Here's how the part is built. I have some questions about the finished solid (model axes, mm). A direction names the side the tool comes from. Give positions to 0.01 mm unless a question says otherwise; leave off trailing zeros. Loops run counter-clockwise (first coordinate to the right, second up) from the corner with the lowest first, then second, coordinate; pieces in that order, holes last. Notation, with made-up numbers: (36, 12) - (87, 12) arc R28 ccw to (87, 34) - close; hole circle Ø5 at (73.25, 73). An arc over 180 degrees is marked (long way). Use a Markdown table: item, result.
from build123d import *

# Parameters (mm, degrees)
F1_DEPTH = 5


with BuildPart() as f1:
    # F0 (on Front) → F1 (new body)
    with BuildSketch(Plane.XZ):
        with BuildLine():
            ThreePointArc((40, 105), (37.071068, 112.071068), (30, 115))
            Line((30, 115), (-30, 115))
            ThreePointArc((-30, 115), (-37.071068, 112.071068), (-40, 105))
            Line((-40, 105), (-40, 97.5))
            Line((-40, 97.5), (-33, 97.5))
            ThreePointArc((-33, 97.5), (-27.87868, 99.62132), (-30, 94.5))
            Line((-30, 94.5), (-30, -94.5))
            ThreePointArc((-30, -94.5), (-27.87868, -99.62132), (-33, -97.5))
            Line((-33, -97.5), (-40, -97.5))
            Line((-40, -97.5), (-40, -105))
            ThreePointArc((-40, -105), (-37.071068, -112.071068), (-30, -115))
            Line((-30, -115), (30, -115))
            ThreePointArc((30, -115), (37.071068, -112.071068), (40, -105))
            Line((40, -105), (40, -97.5))
            Line((40, -97.5), (33, -97.5))
            ThreePointArc((33, -97.5), (27.87868, -99.62132), (30, -94.5))
            Line((30, -94.5), (30, 94.5))
            ThreePointArc((30, 94.5), (27.87868, 99.62132), (33, 97.5))
            Line((33, 97.5), (40, 97.5))
            Line((40, 97.5), (40, 105))
        make_face()
    extrude(amount=F1_DEPTH)


solid = f1.part
(1) We'd pull the mould along X, two halves only. Please class faces 1 (the face through (27.95, -2.46, -99.69)), 2 (the face through (-30, -2, 1)), 3 (the face through (-1, -5, 2)): pulls with the +X half, pulls with the -X half, needs draft (parallel to the pull), parting line crosses it, or undercut.
A:
| item | result |
|---|---|
| face 1 | undercut |
| face 2 | pulls with the -X half |
| face 3 | needs draft |
(2) On a 3-axis mill with a long thin cutter (end or side, diameter ignored), from which of +Z, -Z, +X, -X, +Y, -Y can I reach the whole of each face in a straight line? I mean faces 4 (the face through (-36, -2, -97.5)), 5 (the face through (36, -2, 97.5)), 6 (the face through (-27.95, -2.46, 99.69)). Say none if no direction works.
A:
| item | result |
|---|---|
| face 4 | -X, +Y, -Y |
| face 5 | +X, +Y, -Y |
| face 6 | +Y, -Y |
(3) If I drill on line 1 (Z direction, x = -30.5, y = -3); line 2 (X direction, y = -2.3, z = -15.5); line 3 (Z direction, x = 32, y = -4.65), over which ranges is the centre line in solid material (lowest first)?
A:
| item | result |
|---|---|
| line 1 | -114.99 to -100.46, 100.46 to 114.99 |
| line 2 | -30 to 30 |
| line 3 | -114.8 to -99.74, 99.74 to 114.8 |
(4) Will these pins go through, and if not, where does the flat tip stop? pin 1 (1.5 mm diameter, centred on x = -38, y = -2.5, fed in from -Z); pin 2 (1 mm diameter, centred on y = -1, z = -37, fed in from -X); pin 3 (2.5 mm diameter, centred on x = -37.5, y = -3.5, fed in from +Z).
A:
| item | result |
|---|---|
| pin 1 | z = -111.89 |
| pin 2 | x = -30 |
| pin 3 | z = 112.81 |
(5) Suppose I cut it at A-A on y = -4.1. Write out the boundary of the cut face in (x, z), plus the area to 3 significant figures.
A:
| item | result |
|---|---|
| outline | (-40, -105) arc R10 ccw to (-30, -115) - (30, -115) arc R10 ccw to (40, -105) - (40, -97.5) - (33, -97.5) arc R3 cw (long way) to (30, -94.5) - (30, 94.5) arc R3 cw (long way) to (33, 97.5) - (40, 97.5) - (40, 105) arc R10 ccw to (30, 115) - (-30, 115) arc R10 ccw to (-40, 105) - (-40, 97.5) - (-33, 97.5) arc R3 cw (long way) to (-30, 94.5) - (-30, -94.5) arc R3 cw (long way) to (-33, -97.5) - (-40, -97.5) - close |
| area | 14,300 mm2 |
(6) Suppose I cut it at B-B on z = -91.5. Write out the boundary of the cut face in (x, y).
A:
| item | result |
|---|---|
| outline | (-30, -5) - (30, -5) - (30, 0) - (-30, 0) - close |
